```python
from build123d import *

# Parameters (mm, degrees)
F0_W     = 237.0582
F0_H     = 914.4
F0_R     = 1.575
F0_W_2   = 173.5582
F0_H_2   = 285.75
F1_DEPTH = 2.032


with BuildPart() as f1:
    # F0 (on Top) → F1 (new body)
    with BuildSketch(Plane.XY):
        with Locations((-350.303008, -0.575709)):
            Rectangle(F0_W, F0_H)
        with Locations((-462.482108, -451.425709)):
            Circle(F0_R, mode=Mode.SUBTRACT)
        with Locations((-462.482108, -301.142376)):
            Circle(F0_R, mode=Mode.SUBTRACT)
        with Locations((-462.482108, -150.859042)):
            Circle(F0_R, mode=Mode.SUBTRACT)
        with Locations((-350.303008, -451.425709)):
            Circle(F0_R, mode=Mode.SUBTRACT)
        with Locations((-350.303008, -289.500709)):
            Rectangle(F0_W_2, F0_H_2, mode=Mode.SUBTRACT)
        with Locations((-238.123908, -451.425709)):
            Circle(F0_R, mode=Mode.SUBTRACT)
        with Locations((-238.123908, -301.142376)):
            Circle(F0_R, mode=Mode.SUBTRACT)
        with Locations((-238.123908, -150.859042)):
            Circle(F0_R, mode=Mode.SUBTRACT)
        with Locations((-462.482108, -0.575709)):
            Circle(F0_R, mode=Mode.SUBTRACT)
        with Locations((-462.482108, 149.707624)):
            Circle(F0_R, mode=Mode.SUBTRACT)
        with Locations((-462.482108, 299.990958)):
            Circle(F0_R, mode=Mode.SUBTRACT)
        with Locations((-462.482108, 450.274291)):
            Circle(F0_R, mode=Mode.SUBTRACT)
        with Locations((-238.123908, -0.575709)):
            Circle(F0_R, mode=Mode.SUBTRACT)
        with Locations((-238.123908, 149.707624)):
            Circle(F0_R, mode=Mode.SUBTRACT)
        with Locations((-350.303008, 288.349291)):
            Rectangle(F0_W_2, F0_H_2, mode=Mode.SUBTRACT)
        with Locations((-350.303008, 450.274291)):
            Circle(F0_R, mode=Mode.SUBTRACT)
        with Locations((-238.123908, 299.990958)):
            Circle(F0_R, mode=Mode.SUBTRACT)
        with Locations((-238.123908, 450.274291)):
            Circle(F0_R, mode=Mode.SUBTRACT)
    extrude(amount=F1_DEPTH)


solid = f1.part
```
CAD build for the part. Positions are in the model's coordinates, mm. Round coordinates to 2 decimals unless told otherwise and drop trailing zeros. Loops run counter-clockwise (first coordinate to the right, second up) from the corner with the lowest first, then second, coordinate; pieces in that order, holes last. Notation, with made-up numbers: M -0.5,71.25 L 53.5,71.25 A32 ccw 53.5,110.25 Z; hole C -26.5,45 d4. An arc over 180 degrees is marked long. Use a Markdown table: item, result. Add a question column.
(1) Pull direction Z, two halves, no side cores. Call faces 1 (the face through (-352, 6, 0)), 2 (the face through (-352, 6, 2.032)): +Z half, -Z half, draft (parallel to the pull), parting line (faces both ways), or undercut.
(2) Cut at A-A (x = -276.5). Give the cut face in (y, z).
(3) Drill centre lines: line 1 (Y direction, x = -310, z = 1.75); line 2 (X direction, y = 287, z = 0.55). Where is each one in solid material? Low to high.
(4) Cut at B-B (z = 1.4). State how many separate pieces and enclosed holes the cut face has, and give its area (3 significant figures).
(5) Flat gauge pin, fed straight in: pin 1 (3 mm diameter, centred on x = -238.12, y = 299.99, fed in from -Z). Where does the tip first touch, or does it go through?
Geometry says:
| question | item | result |
|---|---|---|
| 1 | face 1 | -Z half |
| 1 | face 2 | +Z half |
| 2 | outline | M -457.78,0 L -432.38,0 L -432.38,2.03 L -457.78,2.03 Z; M -146.63,0 L 145.47,0 L 145.47,2.03 L -146.63,2.03 Z; M 431.22,0 L 456.62,0 L 456.62,2.03 L 431.22,2.03 Z |
| 3 | line 1 | y = -457.78 to -432.38, -146.63 to 145.47, 431.22 to 456.62 |
| 3 | line 2 | x = -468.83 to -437.08, -263.52 to -231.77 |
| 4 | separate pieces | 1 |
| 4 | enclosed holes | 18 |
| 4 | area | 117,000 mm² |
| 5 | pin 1 | passes through |
